Check sheet for the modelled part. Datum: model origin and axes. Units: mm. A direction names the side the tool comes from. Round coordinates to 2 decimals unless told otherwise and drop trailing zeros. Loops run counter-clockwise (first coordinate to the right, second up) from the corner with the lowest first, then second, coordinate; pieces in that order, holes last. Notation, with made-up numbers: (65.25, 87) -> (123.25, 87) arc R17 cw to (123.25, 99) -> close; hole circle Ø5 at (46, 37). An arc over 180 degrees is marked (long way). Return JSON: item names as keys, results as strings.
from build123d import *

# Parameters (mm, degrees)
CROQUIS1_W                   = 360
CROQUIS1_H                   = 225
SALIENTE_EXTRUIR1_DEPTH      = 135
SALIENTE_EXTRUIR1_DEPTH_BACK = 135
VACIADO1_T                   = -4


with BuildPart() as part:
    # Croquis1 → Saliente-Extruir1 (new body, two sides)
    with BuildSketch(Plane.XY) as saliente_extruir1_sk:
        Rectangle(CROQUIS1_W, CROQUIS1_H)
    extrude(amount=SALIENTE_EXTRUIR1_DEPTH)
    extrude(saliente_extruir1_sk.sketch, amount=-SALIENTE_EXTRUIR1_DEPTH_BACK)

    # Vaciado1
    vaciado1_openings = [part.faces().sort_by_distance(p)[0] for p in [
        (0, 112.5, 0),
    ]]
    offset(amount=VACIADO1_T, openings=vaciado1_openings, kind=Kind.INTERSECTION)


solid = part.part
Q1. Go/stop test with a flat-tipped pin: pin 1 (6 mm diameter, centred on x = -4.5, z = 51.5, fed in from +Y). Record where the tip stops, or that it passes through.
Results list:
{"pin 1": "y = -108.5"}
Q2. Material ranges on line 1 (X direction, y = 2, z = -52.5); line 2 (Z direction, x = -70.5, y = 103); line 3 (Y direction, x = 165, z = 38.5), recorded low to high.
Results list:
{"line 1": "-180 to -176, 176 to 180", "line 2": "-135 to -131, 131 to 135", "line 3": "-112.5 to -108.5"}
Q3. Draft check along Z on faces 3 (the flat face through (-2, 4, 131)), 4 (the flat face through (-3, 2, -135)), 5 (the flat face through (-2, -108.5, 2)), 6 (the flat face through (180, -2, 2)). Enter one of: released by +Z, released by -Z, zero draft, split by the parting line, or undercut.
Results list:
{"face 3": "undercut", "face 4": "released by -Z", "face 5": "undercut", "face 6": "zero draft"}
Q4. Section check C-C (z = -24.5). Record the boundary of the cut face in (x, y), then the cut area to 3 significant figures.
Results list:
{"outline": "(-180, -112.5) -> (180, -112.5) -> (180, 112.5) -> (176, 112.5) -> (176, -108.5) -> (-176, -108.5) -> (-176, 112.5) -> (-180, 112.5) -> close", "area": "3,210 mm^2"}
Q5. Tool access check on faces 1 (the flat face through (-2, 4, -131)), 2 (the flat face through (-3, 2, 135)). Record the directions out of +Z, -Z, +X, -X, +Y, -Y that give a thin tool (end or side, any length) a straight path to the whole face; none if there is none.
Results list:
{"face 1": "+Y", "face 2": "+Z, +X, -X, +Y, -Y"}
Q6. Section check B-B (x = 37.5). Record the boundary of the cut face in (y, z).
Results list:
{"outline": "(-112.5, -135) -> (112.5, -135) -> (112.5, -131) -> (-108.5, -131) -> (-108.5, 131) -> (112.5, 131) -> (112.5, 135) -> (-112.5, 135) -> close"}
Q7. Section check A-A (y = 38). Record the boundary of the cut face in (x, z).
Results list:
{"outline": "(-180, -135) -> (180, -135) -> (180, 135) -> (-180, 135) -> close; hole (-176, -131) -> (176, -131) -> (176, 131) -> (-176, 131) -> close"}
